Part model, mm, in its own coordinate system. Face numbers are marked on the shaded views. A direction names the side the tool comes from. Coordinates: 2 decimals unless noted, no trailing zeros. Order: outer loops, then holes, each group sorted by start corner. A loop starts at its lowest first (then second) coordinate and runs counter-clockwise, first axis right, second up.
1) Cut at B-B (y = 15.5). List the corners of the cut face in (x, z), and give its area (3 significant figures).
2) Cut at A-A (z = -1.5). List the corners of the cut face in (x, y).
3) Pin check, flat tips, straight feed: pin 1 Ø5 at (x, z) = (-17, 5.5) entering from +Y; pin 2 Ø4.5 at (x, z) = (-16.5, -2) entering from -Y; pin 3 Ø15.5 at (x, z) = (-14, 30.5) entering from -Y; pin 4 Ø22 at (x, y) = (-17, 36.5) entering from +Z. Stop position of each tip, or through.
4) Cut at D-D (x = -9). Give the number of separate pieces and of enclosed holes in the cut face, and give its area (3 significant figures).
5) Wall check: L1, parallel to Y at x = -36, z = 2.5; L2, parallel to Z at x = -9, y = 6.3; L3, parallel to Y at x = -5, z = -35.5. Give the ranges that are in metal, low to high.
6) Mould opens along Y. For the marked faces 1, 2, 3 and 4 say: +Y half, -Y half, draft (parallel to the pull), parting line (faces both ways), or undercut.
7) Tool access for the marked faces 5, 6, 7, 8 and 9: list every direction of +Z, -Z, +X, -X, +Y, -Y with a clear straight run to the whole face (end or side of a thin tool).
```python
from build123d import *

# Parameters (mm, degrees)
SKETCH4_R               = 48.26
BOSS_EXTRUDE2_DEPTH     = 40
CUT_EXTRUDE1_DEPTH      = 41
CIRPATTERN1_COUNT       = 4
CUT_EXTRUDE2_DEPTH      = 40
CUT_EXTRUDE3_START      = -3
SKETCH7_R               = 3.5
CUT_EXTRUDE3_DEPTH      = 15
CUT_EXTRUDE4_START      = -3
SKETCH8_R               = 3.5
CUT_EXTRUDE4_DEPTH      = 15
CUT_EXTRUDE5_START      = -3.062685
SKETCH11_R              = 2.38125
CUT_EXTRUDE5_DEPTH      = 3.062685
SKETCH13_R              = 2.38125
CUT_EXTRUDE6_DEPTH      = 68.952595383
CUT_EXTRUDE6_DEPTH_BACK = 68.952595383


with BuildPart() as part:
    # Sketch4 → Boss-Extrude2 (new body)
    with BuildSketch(Plane(origin=(0, 0, 0), x_dir=(0, 0, -1), z_dir=(1, 0, 0))):
        Circle(SKETCH4_R)
    extrude(amount=-BOSS_EXTRUDE2_DEPTH)

    # Sketch6 → Cut-Extrude1 (cut, through all)
    with BuildSketch(Plane(origin=(0, 0, 0), x_dir=(0, 0, -1), z_dir=(1, 0, 0))):
        Polygon((-4.5, 277.678371005), (-4.5, 48.049740894), (-4.5, 28.049740894), (4.5, 28.049740894), (4.5, 48.049740894), (4.5, 277.678371005), (4.5, 736.935631227), (-4.5, 736.935631227), align=None)
    cut_extrude1 = extrude(amount=-CUT_EXTRUDE1_DEPTH, mode=Mode.SUBTRACT)

    # CirPattern1: Cut-Extrude1 ×4 about axis
    cirpattern1_axis = Axis((0, 0, 0), (1, 0, 0))
    for i in range(1, CIRPATTERN1_COUNT):
        add(cut_extrude1.rotate(cirpattern1_axis, i * 360 / CIRPATTERN1_COUNT), mode=Mode.SUBTRACT)

    # Sketch9 → Cut-Extrude2 (cut)
    with BuildSketch(Plane(origin=(0, 0, 0), x_dir=(0, 0, -1), z_dir=(1, 0, 0))):
        with BuildLine():
            Line((-25.049740894, -7.5), (-44.634264865, -7.5))
            ThreePointArc((-44.634264865, -7.5), (-32.003652917, -32.003652917), (-7.5, -44.634264865))
            Line((-7.5, -44.634264865), (-7.5, -25.049740894))
            Line((-7.5, -25.049740894), (7.5, -25.049740894))
            Line((7.5, -25.049740894), (7.5, -44.634264865))
            ThreePointArc((7.5, -44.634264865), (32.003652917, -32.003652917), (44.634264865, -7.5))
            Line((44.634264865, -7.5), (25.049740894, -7.5))
            Line((25.049740894, -7.5), (25.049740894, 7.5))
            Line((25.049740894, 7.5), (44.634264865, 7.5))
            ThreePointArc((44.634264865, 7.5), (32.003652917, 32.003652917), (7.5, 44.634264865))
            Line((7.5, 44.634264865), (7.5, 25.049740894))
            Line((7.5, 25.049740894), (-7.5, 25.049740894))
            Line((-7.5, 25.049740894), (-7.5, 44.634264865))
            ThreePointArc((-7.5, 44.634264865), (-32.003652917, 32.003652917), (-44.634264865, 7.5))
            Line((-44.634264865, 7.5), (-25.049740894, 7.5))
            Line((-25.049740894, 7.5), (-25.049740894, -7.5))
        make_face()
    extrude(amount=-CUT_EXTRUDE2_DEPTH, mode=Mode.SUBTRACT)

    # Sketch7 → Cut-Extrude3 (cut)
    with BuildSketch(Plane.XY.offset(-4.5).offset(CUT_EXTRUDE3_START)):
        with Locations((-9, 37.049740894)):
            Circle(SKETCH7_R)
    cut_extrude3 = extrude(amount=CUT_EXTRUDE3_DEPTH, mode=Mode.SUBTRACT)

    # Sketch8 → Cut-Extrude4 (cut)
    with BuildSketch(Plane.XZ.offset(-4.5).offset(CUT_EXTRUDE4_START)):
        with Locations((-9, 37.049740894)):
            Circle(SKETCH8_R)
    cut_extrude4 = extrude(amount=CUT_EXTRUDE4_DEPTH, mode=Mode.SUBTRACT)

    # Mirror1: Cut-Extrude3 across plane
    add(cut_extrude3.mirror(Plane.ZX), mode=Mode.SUBTRACT)

    # Mirror2: Cut-Extrude4 across plane
    add(cut_extrude4.mirror(Plane.XY), mode=Mode.SUBTRACT)

    # Sketch11 → Cut-Extrude5 (cut)
    with BuildSketch(Plane(origin=(0, -34.12497326, 34.12497326), x_dir=(1, 0, 0), z_dir=(0, -0.707106781, 0.707106781)).offset(CUT_EXTRUDE5_START)):
        with Locations((-20, 0)):
            Circle(SKETCH11_R)
    cut_extrude5 = extrude(amount=CUT_EXTRUDE5_DEPTH, mode=Mode.SUBTRACT)

    # Mirror3: Cut-Extrude5 across plane
    add(cut_extrude5.mirror(Plane(origin=(0, 0, 0), x_dir=(0, 0.707106781, 0.707106781), z_dir=(0, 0.707106781, -0.707106781))), mode=Mode.SUBTRACT)

    # Sketch13 → Cut-Extrude6 (cut, two sides)
    with BuildSketch(Plane(origin=(0, 0, 0), x_dir=(1, 0, 0), z_dir=(0, 0.707106781, 0.707106781))) as cut_extrude6_sk:
        with Locations((-20, 0)):
            Circle(SKETCH13_R)
    extrude(amount=CUT_EXTRUDE6_DEPTH, mode=Mode.SUBTRACT)
    extrude(cut_extrude6_sk.sketch, amount=-CUT_EXTRUDE6_DEPTH_BACK, mode=Mode.SUBTRACT)


solid = part.part
```
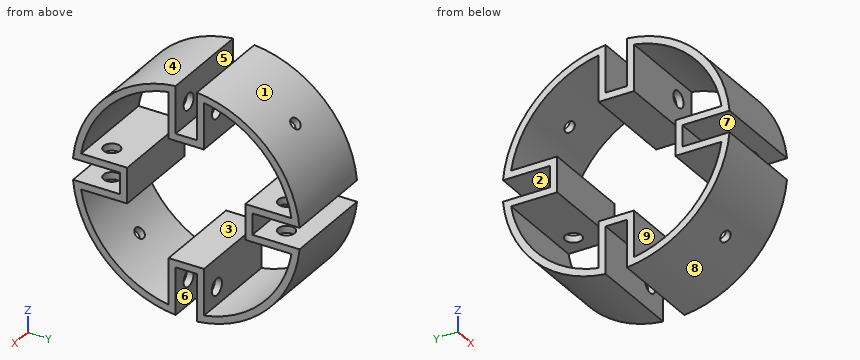
Geometry check:
1. outline: (-40, -45.7) - (0, -45.7) - (0, -42.52) - (-40, -42.52) - close; (-40, 42.52) - (0, 42.52) - (0, 45.7) - (-40, 45.7) - close
1. area: 254 mm2
2. outline: (-40, -28.05) - (0, -28.05) - (0, -25.05) - (-40, -25.05) - close; (-40, 25.05) - (0, 25.05) - (0, 28.05) - (-40, 28.05) - close
3. pin 1: stops at y = 48.05
3. pin 2: stops at y = -28.05
3. pin 3: stops at y = -42.56
3. pin 4: stops at z = 40.97
4. separate pieces: 8
4. enclosed holes: 0
4. area: 1,190 mm2
5. L1: y = -28.05 to -25.05, 25.05 to 28.05
5. L2: z = -47.85 to -40.55, -33.55 to -25.05, 25.05 to 33.55, 40.55 to 47.85
5. L3: y = -32.69 to -28.08, -7.5 to -4.5, 4.5 to 7.5, 28.08 to 32.69
6. face 1: +Y half
6. face 2: draft
6. face 3: undercut
6. face 4: -Y half
7. face 5: +Z, +X, -X
7. face 6: -Z, +X, -X
7. face 7: +X, -X, -Y
7. face 8: -Z, +X, -X, -Y
7. face 9: +X, -X
